For this review, take the finished solid that the model builds, in its own axes (mm). A direction names the side the tool comes from. Round coordinates to 2 decimals unless told otherwise and drop trailing zeros. Order: outer loops, then holes, each group sorted by start corner. A loop starts at its lowest first (then second) coordinate and runs counter-clockwise, first axis right, second up. Notation, with made-up numbers: (35, 63) - (70, 63) arc R5 ccw to (70, 70) - close; hole circle Ø2 at (12, 41.5). An arc over 180 degrees is marked (long way). One line per item, written item: value.
```python
from build123d import *

# Parameters (mm, degrees)
EXTRUDE_1_DEPTH      = 9
EXTRUDE_1_DEPTH_BACK = 9
EXTRUDE_2_DEPTH      = 6
EXTRUDE_2_DEPTH_BACK = 6
EXTRUDE_3_DEPTH      = 4
EXTRUDE_3_DEPTH_BACK = 4
FILLET_2_R           = 2


with BuildPart() as part:
    # 草图1 → 凸台-拉伸1 (new, two sides: drawn at the far end of the back side and taken through both)
    with BuildSketch(Plane(origin=(0, 0, 0), x_dir=(0, 0, -1), z_dir=(1, 0, 0)).offset(-EXTRUDE_1_DEPTH_BACK)):
        Polygon((0, 17.5), (0, 40), (42.5, 40), (42.5, 22.5), (65.5, 22.5), (65.5, -22.5), (42.5, -22.5), (42.5, -40), (0, -40), (0, -17.5), (5.084959992, -17.5), (5.084959992, 17.5), align=None)
    extrude(amount=EXTRUDE_1_DEPTH + EXTRUDE_1_DEPTH_BACK)

    # 草图2 → 凸台-拉伸2 (add, two sides: drawn at the far end of the back side and taken through both)
    with BuildSketch(Plane(origin=(0, 0, 0), x_dir=(0, 0, -1), z_dir=(1, 0, 0)).offset(-EXTRUDE_2_DEPTH_BACK)):
        with BuildLine():
            Line((65.5, -3.307764834), (65.5, -13.668635082))
            ThreePointArc((65.5, -13.668635082), (70.680435124, -8.488199958), (65.5, -3.307764834))
        make_face()
    extrude(amount=EXTRUDE_2_DEPTH + EXTRUDE_2_DEPTH_BACK)

    # 草图3 → 凸台-拉伸3 (add, two sides: drawn at the far end of the back side and taken through both)
    with BuildSketch(Plane(origin=(0, 0, 0), x_dir=(0, 0, -1), z_dir=(1, 0, 0)).offset(-EXTRUDE_3_DEPTH_BACK)):
        Polygon((69.816037918, -8.168812248), (67.126357089, -12.498830138), (75.576408791, -17.747755811), (78.26608962, -13.41773792), align=None)
    extrude(amount=EXTRUDE_3_DEPTH + EXTRUDE_3_DEPTH_BACK)

    # 圆角2
    fillet_2_edges = [part.edges().sort_by_distance(p)[0] for p in [
        (0, -17.747755811, -75.576408791),
        (0, -13.41773792, -78.26608962),
    ]]
    fillet(fillet_2_edges, radius=FILLET_2_R)


solid = part.part
```
Item 1: Take a section at D-D (x = 7.25). Write out the cut boundary in (y, z), plus the area to 3 significant figures.
Returned:
outline: (-40, -42.5) - (-22.5, -42.5) - (-22.5, -65.5) - (22.5, -65.5) - (22.5, -42.5) - (40, -42.5) - (40, 0) - (17.5, 0) - (17.5, -5.08) - (-17.5, -5.08) - (-17.5, 0) - (-40, 0) - close
area: 4,260 mm^2
Item 2: Take a section at C-C (y = -1.5). Write out the cut boundary in (x, z), plus the area to 3 significant figures.
Returned:
outline: (-9, -65.5) - (9, -65.5) - (9, -5.08) - (-9, -5.08) - close
area: 1,090 mm^2
Item 3: For P1, Ø4, axis at y = -11.5, z = -74, coming from the +X side; P2, Ø1.5, axis at x = 3, y = -17, coming from the -Z side; P3, Ø9, axis at x = -1.5, z = -56.5, coming from the +Y side, all flat-tipped, find the tip position at first contact; note any pin that passes through.
Returned:
P1: x = 4
P2: z = -76.49
P3: y = 22.5
Item 4: Wall thickness on line 1 (Y direction, x = 7.5, z = -57); line 2 (Y direction, x = 5, z = -4.5); line 3 (Z direction, x = -7.25, y = -24): over which ranges is each line inside the solid? List them lowest first.
Returned:
line 1: -22.5 to 22.5
line 2: -40 to -17.5, 17.5 to 40
line 3: -42.5 to 0
Item 5: Machinability: for faces 1 (the flat face through (0, -22.5, -54)), 2 (the flat face through (-6, -8, -67)), 3 (the flat face through (0, 0, -5.085)), 4 (the flat face through (0, 22.5, -54)), which of the approach directions +Z, -Z, +X, -X, +Y, -Y give a long, thin tool a straight path to every point of the face, cutting with its end or side? Answer none if there is none.
Returned:
face 1: -Z, +X, -X, -Y
face 2: -Z, -X, +Y, -Y
face 3: +Z, +X, -X
face 4: -Z, +X, -X, +Y
Item 6: The part is to be moulded in two halves that separate along Z. For faces 5 (the flat face through (9, 1, -33)), 6 (the cylindrical face through (0.056, -16.936, -75.409)), 7 (the flat face through (0, -31, -42.5)), say which applies: +Z half, -Z half, draft (parallel to the pull), parting line (faces both ways), or undercut.
Returned:
face 5: draft
face 6: undercut
face 7: -Z half
Item 7: Take a section at A-A (x = -5). Write out the cut boundary in (y, z).
Returned:
outline: (-40, -42.5) - (-22.5, -42.5) - (-22.5, -65.5) - (-13.67, -65.5) arc R5.18 ccw to (-3.31, -65.5) - (22.5, -65.5) - (22.5, -42.5) - (40, -42.5) - (40, 0) - (17.5, 0) - (17.5, -5.08) - (-17.5, -5.08) - (-17.5, 0) - (-40, 0) - close
Item 8: Take a section at B-B (z = -69.5). Write out the cut boundary in (x, y), plus the area to 3 significant figures.
Returned:
outline: (-6, -11.78) - (-4, -11.78) - (-4, -13.97) - (4, -13.97) - (4, -11.78) - (6, -11.78) - (6, -5.2) - (-6, -5.2) - close
area: 96.6 mm^2
